Model file for the job. Use its own axes, mm. Round coordinates to 2 decimals unless told otherwise and drop trailing zeros. Use one line per item in the form item = value.
from build123d import *

# Parameters (mm, degrees)
SKETCH1_R           = 8.5
SKETCH1_R_2         = 2.55
BOSS_EXTRUDE1_DEPTH = 7
BOSS_EXTRUDE2_START = 7
SKETCH1_3_R         = 8.5
SKETCH1_3_R_2       = 2.55
BOSS_EXTRUDE2_DEPTH = 4
CHAMFER1_SIZE       = 2
FILLET2_R           = 2
CUT_EXTRUDE1_START  = -9
SKETCH2_R           = 5.25
CUT_EXTRUDE1_DEPTH  = 2


with BuildPart() as part:
    # Sketch1 → Boss-Extrude1 (new body)
    with BuildSketch(Plane.XY):
        with BuildLine():
            ThreePointArc((92.127210642, -71.744668074), (53.839787702, -31.020916727), (0, -16))
            ThreePointArc((0, -16), (-16, 0), (0, 16))
            ThreePointArc((0, 16), (70.405876226, -3.642737258), (120.474044686, -56.896873635))
            ThreePointArc((120.474044686, -56.896873635), (113.724524883, -78.494187876), (92.127210642, -71.744668074))
        make_face()
        Circle(SKETCH1_R, mode=Mode.SUBTRACT)
        with BuildLine():
            ThreePointArc((112.501497611, -61.072815821), (77.057279191, -19.048646747), (27.173726746, 4.058810952))
            ThreePointArc((27.173726746, 4.058810952), (18.838075062, -1.2813118), (24.178197814, -9.616963484))
            ThreePointArc((24.178197814, -9.616963484), (68.562775973, -30.177142381), (100.099757717, -67.568725888))
            ThreePointArc((100.099757717, -67.568725888), (109.548582697, -70.521640801), (112.501497611, -61.072815821))
        make_face(mode=Mode.SUBTRACT)
        Circle(SKETCH1_R)
        Circle(SKETCH1_R_2, mode=Mode.SUBTRACT)
    extrude(amount=BOSS_EXTRUDE1_DEPTH)

    # Sketch1<3> → Boss-Extrude2 (add)
    with BuildSketch(Plane.XY.offset(BOSS_EXTRUDE2_START)):
        Circle(SKETCH1_3_R)
        Circle(SKETCH1_3_R_2, mode=Mode.SUBTRACT)
    extrude(amount=BOSS_EXTRUDE2_DEPTH)

    # Chamfer1
    chamfer1_edges = [part.edges().sort_by_distance(p)[0] for p in [
        (113.724524883, -78.494187876, 7),
        (18.838075062, -1.2813118, 0),
        (68.562775973, -30.177142381, 0),
        (109.548582697, -70.521640801, 0),
        (77.057279191, -19.048646747, 0),
        (-16, 0, 0),
        (70.405876226, -3.642737258, 0),
        (113.724524883, -78.494187876, 0),
        (70.405876226, -3.642737258, 7),
        (53.839787702, -31.020916727, 0),
        (-16, 0, 7),
        (77.057279191, -19.048646747, 7),
        (109.548582697, -70.521640801, 7),
        (68.562775973, -30.177142381, 7),
        (18.838075062, -1.2813118, 7),
        (53.839787702, -31.020916727, 7),
    ]]
    chamfer(chamfer1_edges, length=CHAMFER1_SIZE)

    # Fillet2
    fillet2_edges = [part.edges().sort_by_distance(p)[0] for p in [
        (-8.5, 0, 7),
    ]]
    fillet(fillet2_edges, radius=FILLET2_R)

    # Sketch2 → Cut-Extrude1 (cut)
    with BuildSketch(Plane.XY.offset(11).offset(CUT_EXTRUDE1_START)):
        Circle(SKETCH2_R)
    extrude(amount=-CUT_EXTRUDE1_DEPTH, mode=Mode.SUBTRACT)


solid = part.part
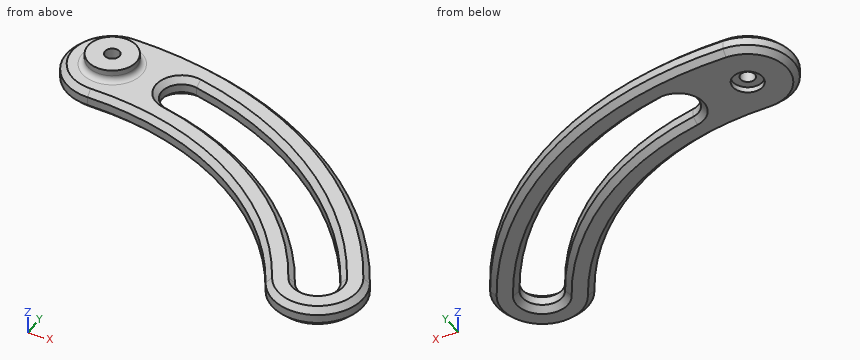
1. Flat gauge pins, fed straight in: pin 1 (2 mm diameter, centred on x = 78.5, z = 7, fed in from -Y); pin 2 (1.5 mm diameter, centred on x = 45.5, z = 6.5, fed in from +Y); pin 3 (1.5 mm diameter, centred on y = -8, z = 9, fed in from +X). Where does each tip first touch, or does it go through?
Geometry check:
pin_1 = -50.64
pin_2 = 7.41
pin_3 = 4.44
2. Wall check: probe 1 along Y at (x, z) = (0, 9.25); probe 2 along Y at (x, z) = (0, 0.5); probe 3 along Z at (x, y) = (40, -20.5). Give the ranges that are in metal, low to high.
Geometry check:
probe_1 = -8.5 to -2.55, 2.55 to 8.5
probe_2 = -14.5 to -5.25, 5.25 to 14.5
probe_3 = 0 to 7
3. Cut at A-A, the plane y = 0. Give the number of separate pieces and of enclosed holes in the cut face, plus the area to 3 significant figures.
Geometry check:
separate_pieces = 3
enclosed_holes = 0
area = 378 mm^2
